Check sheet for the modelled part. Datum: model origin and axes. Units: mm. Face numbers are marked on the shaded views. A direction names the side the tool comes from. Give positions to 0.01 mm unless a question says otherwise; leave off trailing zeros. Loops run counter-clockwise (first coordinate to the right, second up) from the corner with the lowest first, then second, coordinate; pieces in that order, holes last. Notation, with made-up numbers: M 17.25,-38.75 L 38.25,-38.75 A28 ccw 38.25,-15.75 Z; hole C 53,-36 d9. An arc over 180 degrees is marked long. Write each question's results on one line, items separated by ' | '. Start each with the question number.
1. Tool access check on the marked faces 4, 5, 6 and 7. Record the directions out of +Z, -Z, +X, -X, +Y, -Y that give a thin tool (end or side, any length) a straight path to the whole face; none if there is none.
2. Go/stop test with flat-tipped pins: pin 1 (8 mm diameter, centred on x = 6.5, y = 20.5, fed in from -Z); pin 2 (0.9 mm diameter, centred on x = 5, y = 10, fed in from +Z); pin 3 (0.8 mm diameter, centred on x = 11.5, y = 15.5, fed in from +Z). Record where each tip stops, or that it passes through.
3. Material ranges on line 1 along Z through (x, y) = (15.25, 29); line 2 along Z through (x, y) = (9.5, 22.5); line 3 along Y through (x, z) = (10.25, 8.5), recorded low to high.
4. Sectioned sample at D-D on y = 26. Record the cut outline in (x, z).
5. Sectioned sample at C-C on z = 13. Record the cut outline in (x, y), and give its area (3 significant figures).
6. Draft check along Y on the marked faces 1, 2 and 3. Enter one of: pulls with the +Y half, pulls with the -Y half, needs draft (parallel to the pull), parting line crosses it, or undercut.
7. Sectioned sample at A-A on y = 13.5. Record the cut outline in (x, z).
```python
from build123d import *

# Parameters (mm, degrees)
F1_DEPTH     = 16
F2_R         = 7.99999
F3_R         = 20
F4_R         = 3.99999
F6_DEPTH     = 34.001
F8_DEPTH     = 4
F11_R        = 1
F12_T1_DEPTH = 33.00001


# Not quite as in the source:
# - a fillet or chamfer that OpenCascade refuses, or shapes differently, is made with other operations: its cross-section is extruded or revolved along the edge and cut away or added
# - a fillet or chamfer is up to 0.001 mm smaller than in the source, because OpenCascade refuses the exact size


with BuildPart() as f1:
    # F0 (on Right) → F1 (new body)
    with BuildSketch(Plane.YZ):
        Polygon((34, 34), (0, 34), (0, 0), (16, 0), (16, 9), (11, 9), (11, 5), (8, 5), (8, 22), (34, 22), align=None)
    extrude(amount=F1_DEPTH)

    # F2 (radius 8 in the source; OpenCascade refuses exactly that, so slightly less here)
    f2_edges = [f1.edges().sort_by_distance(p)[0] for p in [
        (8, 16, 0),
        (8, 0, 0),
    ]]
    fillet(f2_edges, radius=F2_R)

    # F3
    f3_edges = [f1.edges().sort_by_distance(p)[0] for p in [
        (8, 0, 34),
    ]]
    fillet(f3_edges, radius=F3_R)

    # F4 (radius 4 in the source; OpenCascade refuses exactly that, so slightly less here)
    f4_edges = [f1.edges().sort_by_distance(p)[0] for p in [
        (8, 8, 22),
        (8, 11, 9),
    ]]
    fillet(f4_edges, radius=F4_R)

    # F5 (on face) → F6 (cut, through all)
    with BuildSketch(Plane.XY.offset(34)):
        with BuildLine():
            ThreePointArc((1.5, 34), (8, 27.5), (14.5, 34))
            Line((14.5, 34), (1.5, 34))
        make_face()
    extrude(amount=-F6_DEPTH, mode=Mode.SUBTRACT)


with BuildPart() as f8:
    # F7 (on face) → F8 (new body)
    with BuildSketch(Plane.XY.offset(34)):
        with BuildLine():
            ThreePointArc((16, 31.1277186767), (8, 25.5), (0, 31.1277186767))
            Line((0, 31.1277186767), (0, 25.7386441791))
            ThreePointArc((0, 25.7386441791), (8, 22.5), (16, 25.7386441791))
            Line((16, 25.7386441791), (16, 31.1277186767))
        make_face()
    extrude(amount=F8_DEPTH)


with BuildPart() as f8_1:
    # F9: moved
    add(f8.part.moved(Location((0, 0, -8))))


with BuildPart() as f1_1:
    add(f1.part)

    # F10: cut F8
    add(f8_1.part, mode=Mode.SUBTRACT)

    # F11
    f11_edges = [f1_1.edges().sort_by_distance(p)[0] for p in [
        (16, 34, 28),
        (16, 25.738644, 28),
        (0, 34, 28),
        (0, 25.738644, 28),
    ]]
    fillet(f11_edges, radius=F11_R)

    # F12: fillet of radius 4 on 2 edges, made by hand

    # F12_s2 → F12_t1 (cut)
    with BuildSketch(Plane.XY.offset(-2.00001)):
        with BuildLine():
            ThreePointArc((12, 0), (14.8284271247, 1.1715728753), (16, 4))
            Line((16, 4), (16, 0))
            Line((16, 0), (12, 0))
        make_face()
        with BuildLine():
            ThreePointArc((0, 4), (1.1715728753, 1.1715728753), (4, 0))
            Line((4, 0), (0, 0))
            Line((0, 0), (0, 4))
        make_face()
    extrude(amount=F12_T1_DEPTH, mode=Mode.SUBTRACT)


solid = f1_1.part
```
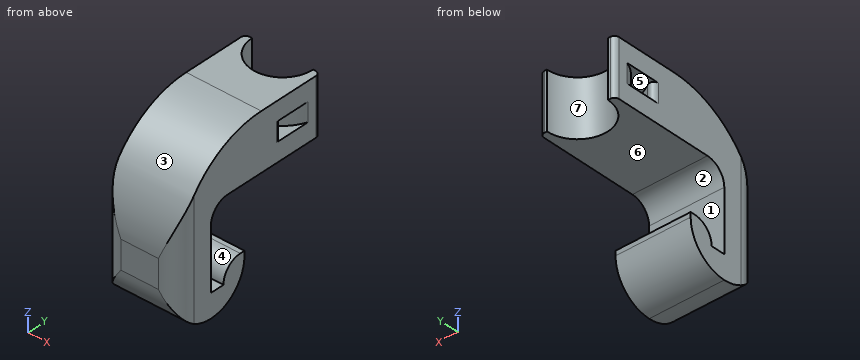
Output values:
1) face 4: +X, -X | face 5: none | face 6: +X, -X, +Y | face 7: +Z, -Z, +Y
2) pin 1: z = 22 | pin 2: z = 31.57 | pin 3: z = 33.58
3) line 1: 22 to 26, 30 to 34 | line 2: 22 to 34 | line 3: 0 to 8, 13.06 to 16
4) outline: M 0,22 L 16,22 L 16,26 L 10.87,26 L 10.87,30 L 16,30 L 16,34 L 0,34 L 0,30 L 5.13,30 L 5.13,26 L 0,26 Z
5) outline: M 0,4 A4 ccw 4,0 L 12,0 A4 ccw 16,4 L 16,8 L 0,8 Z | area: 121 mm2
6) face 1: undercut | face 2: pulls with the +Y half | face 3: pulls with the -Y half
7) outline: M 0,2.19 L 16,2.19 L 16,8.71 L 0,8.71 Z; M 0,22 L 16,22 L 16,32.91 L 0,32.91 Z
